Check sheet for the modelled part. Datum: model origin and axes. Units: mm. A direction names the side the tool comes from. Give positions to 0.01 mm unless a question says otherwise; leave off trailing zeros. Write each loop counter-clockwise with the first axis right and the second up, starting at its lowest first coordinate (ties: lowest second). Pieces come first, ordered by that corner, then holes. Notation, with made-up numbers: (-30.75, 55) -> (21.25, 55) arc R21 cw to (21.25, 79) -> close; hole circle Ø5 at (86.5, -3). An arc over 180 degrees is marked (long way). Use a Markdown table: item, result. Add a question column.
1. Gauge pin test, flat ends, axial feed: P1, Ø1, axis at x = 64.5, y = 6.5, coming from the +Z side; P2, Ø10, axis at y = 5.5, z = 12.5, coming from the -X side; P3, Ø3, axis at x = 36, z = 8, coming from the +Y side. Record the tip position at first contact, or that the pin passes through.
2. Set-up check for faces 1 (the flat face through (15.95, 16, 1)), 2 (the flat face through (49, 0, 4)), 3 (the flat face through (49, 12, 5)): record each of +Z, -Z, +X, -X, +Y, -Y from which the full face is reachable in a straight line by a thin tool's end or side.
3. Cross-section at C-C (y = 15.5). Enter the section's corners in (x, z).
4. Cross-section at A-A (x = 33). Enter the section's corners in (y, z).
5. Release check for a two-part mould opening along X. For faces 4 (the flat face through (95, 12, 12)), 5 (the flat face through (99, 12, 10)), 6 (the flat face through (2, 12, 20)) record: released by +X, released by -X, zero draft, split by the parting line, or undercut.
6. Scan lines: probe 1 along Y at (x, z) = (33, 3.9); probe 2 along X at (y, z) = (19, 2.5); probe 3 along X at (y, z) = (14, 14.5). Record each from-to range of solid material in increasing order. Write a range as [from, to].
7. Cross-section at D-D (y = 2.75). Enter the section's corners in (x, z).
8. Cross-section at B-B (z = 17.25). Enter the section's corners in (x, y).
from build123d import *

# Parameters (mm, degrees)
F0_W     = 91
F0_H     = 24.5
F0_R     = 3
F1_DEPTH = 5
F0_W_2   = 4
F2_DEPTH = 20
F3_R     = 3
F4_DEPTH = 3


with BuildPart() as f1:
    # F0 (on Top) → F1 (new body)
    with BuildSketch(Plane.XY):
        with Locations((49.5, 12.25)):
            Rectangle(F0_W, F0_H)
        with Locations((33, 15.5)):
            Circle(F0_R, mode=Mode.SUBTRACT)
    extrude(amount=F1_DEPTH)

    # F0 (on Top) → F2 (join)
    with BuildSketch(Plane.XY):
        with Locations((2, 12.25)):
            Rectangle(F0_W_2, F0_H)
        with Locations((97, 12.25)):
            Rectangle(F0_W_2, F0_H)
    extrude(amount=F2_DEPTH)

    # F3 (on face) → F4 (cut)
    with BuildSketch(Plane.XY):
        with BuildLine():
            Line((50.05, 22.7), (15.95, 22.7))
            Line((15.95, 22.7), (15.95, 9.3))
            ThreePointArc((15.95, 9.3), (16.242893, 8.592893), (16.95, 8.3))
            Line((16.95, 8.3), (49.05, 8.3))
            ThreePointArc((49.05, 8.3), (49.757107, 8.592893), (50.05, 9.3))
            Line((50.05, 9.3), (50.05, 22.7))
        make_face()
        with Locations((33, 15.5)):
            Circle(F3_R, mode=Mode.SUBTRACT)
    extrude(amount=F4_DEPTH, mode=Mode.SUBTRACT)


solid = f1.part
Worked answers:
| question | item | result |
|---|---|---|
| 1 | P1 | stops at z = 5 |
| 1 | P2 | stops at x = 0 |
| 1 | P3 | passes through |
| 2 | face 1 | -Z |
| 2 | face 2 | +Z, -Z, +X, -X, -Y |
| 2 | face 3 | +Z, +Y, -Y |
| 3 | outline | (0, 0) -> (15.95, 0) -> (15.95, 3) -> (30, 3) -> (30, 5) -> (4, 5) -> (4, 20) -> (0, 20) -> close; (36, 3) -> (50.05, 3) -> (50.05, 0) -> (99, 0) -> (99, 20) -> (95, 20) -> (95, 5) -> (36, 5) -> close |
| 4 | outline | (0, 0) -> (8.3, 0) -> (8.3, 3) -> (12.5, 3) -> (12.5, 5) -> (0, 5) -> close; (18.5, 3) -> (22.7, 3) -> (22.7, 0) -> (24.5, 0) -> (24.5, 5) -> (18.5, 5) -> close |
| 5 | face 4 | undercut |
| 5 | face 5 | released by +X |
| 5 | face 6 | zero draft |
| 6 | probe 1 | y = [0, 12.5], [18.5, 24.5] |
| 6 | probe 2 | x = [0, 15.95], [50.05, 99] |
| 6 | probe 3 | x = [0, 4], [95, 99] |
| 7 | outline | (0, 0) -> (99, 0) -> (99, 20) -> (95, 20) -> (95, 5) -> (4, 5) -> (4, 20) -> (0, 20) -> close |
| 8 | outline | (0, 0) -> (4, 0) -> (4, 24.5) -> (0, 24.5) -> close; (95, 0) -> (99, 0) -> (99, 24.5) -> (95, 24.5) -> close |
